Input: part model. Units: mm. Frame: model coordinates. Give positions to 0.01 mm unless a question says otherwise; leave off trailing zeros. Order: outer loops, then holes, each group sorted by start corner. A loop starts at its lowest first (then second) coordinate and runs counter-clockwise, first axis right, second up. Notation, with made-up numbers: (36.25, -17) -> (85.25, -17) arc R31 cw to (85.25, 15) -> close; hole circle Ø10 at (18.25, 82). An arc over 180 degrees is marked (long way). Use a Markdown table: item, result. Add a question column.
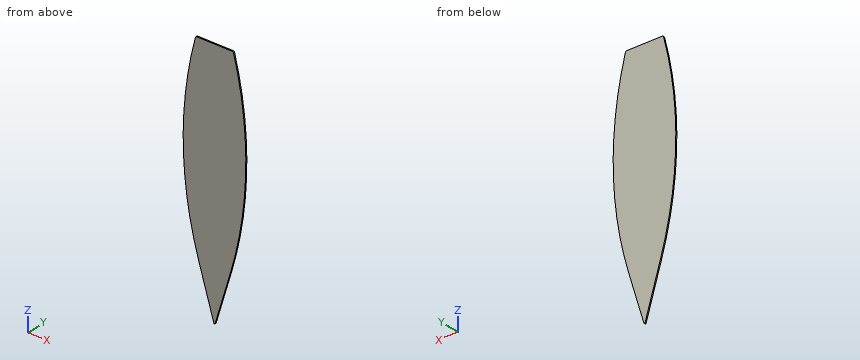
from build123d import *

# Parameters (mm, degrees)
BOSS_EXTRUDE1_DEPTH = 5
FILLET1_R           = 5
FILLET2_R           = 2.5


with BuildPart() as part:
    # Sketch1 → Boss-Extrude1 (new body)
    with BuildSketch(Plane(origin=(0, 0, 0), x_dir=(1, 0, 0), z_dir=(0, 1, 0))):
        with BuildLine():
            Line((-75, -500), (75, -500))
            ThreePointArc((75, -500), (124.853709924, -104.537010412), (63.713442869, 289.338904404))
            Line((63.713442869, 289.338904404), (0, 500))
            Line((0, 500), (-63.713442869, 289.338904404))
            ThreePointArc((-63.713442869, 289.338904404), (-124.853709924, -104.537010412), (-75, -500))
        make_face()
    extrude(amount=BOSS_EXTRUDE1_DEPTH)

    # Fillet1
    fillet1_edges = [part.edges().sort_by_distance(p)[0] for p in [
        (75, 2.5, 500),
        (-75, 2.5, 500),
    ]]
    fillet(fillet1_edges, radius=FILLET1_R)

    # Fillet2
    fillet2_edges = [part.edges().sort_by_distance(p)[0] for p in [
        (0, 2.5, -500),
    ]]
    fillet(fillet2_edges, radius=FILLET2_R)


solid = part.part
Q1. Section query A-A (y = 3.25). Return loops of the section in (x, z), plus the area to 3 significant figures.
Q2. Section query B-B (z = 205). Return loops of the section in (x, y).
Q3. Section query C-C (x = 23.5). Return loops of the section in (y, z), plus the area to 3 significant figures.
Q4. Ray query, line 1 (X direction, y = 0.85, z = -246); line 2 (X direction, y = 3.05, z = -153); line 3 (Z direction, x = 2, y = 4). Return the intervals inside material, ascending.
Q5. First-contact query: pin 1 (8 mm diameter, centred on x = -44, z = -37, fed in from -Y). Flat tip, straight axial feed; report the tip coordinate or a pass-through.
Solution:
| question | item | result |
|---|---|---|
| 1 | outline | (-76, 496.3) arc R1431.25 ccw to (-63.71, -289.34) -> (-2.39, -492.09) arc R2.5 ccw to (2.39, -492.09) -> (63.71, -289.34) arc R1431.25 ccw to (76, 496.3) arc R5 ccw to (71.17, 500) -> (-71.17, 500) arc R5 ccw to start |
| 1 | area | 182,000 mm² |
| 2 | outline | (-122.76, 0) -> (122.76, 0) -> (122.76, 5) -> (-122.76, 5) -> close |
| 3 | outline | (0, -422.3) -> (5, -422.3) -> (5, 500) -> (0, 500) -> close |
| 3 | area | 4,610 mm² |
| 4 | line 1 | x = -76.08 to 76.08 |
| 4 | line 2 | x = -97.74 to 97.74 |
| 4 | line 3 | z = -492.86 to 500 |
| 5 | pin 1 | stops at y = 0 |
